Part model, mm, in its own coordinate system. Face numbers are marked on the shaded views. A direction names the side the tool comes from. Round coordinates to 2 decimals unless told otherwise and drop trailing zeros. Write each loop counter-clockwise with the first axis right and the second up, starting at its lowest first coordinate (ties: lowest second). Pieces come first, ordered by that corner, then holes. Notation, with made-up numbers: M 12.25,34.5 L 25.25,34.5 A27 cw 25.25,61.5 Z; hole C 56.5,43 d10. An arc over 180 degrees is marked long. Answer as a JSON object with one key per item and string values. Group by question number.
1. Band-saw the part on D-D, the plane z = -11. Write the cut outline in (x, y).
2. Band-saw the part on C-C, the plane x = 44. Write the cut outline in (y, z) (1 decimal).
3. Band-saw the part on A-A, the plane y = 6.5. Write the cut outline in (x, z) (1 decimal).
4. Which spindle directions (+Z, -Z, +X, -X, +Y, -Y) get a long thin tool onto all of the face, cutting with end or side? Do the marked faces 1 and 2. Say none if no direction does.
5. Band-saw the part on B-B, the plane z = -29.5. Write the cut outline in (x, y).
6. Drill centre lines: line 1 (X direction, y = 8, z = -43); line 2 (Y direction, x = 39.5, z = -35); line 3 (Z direction, x = 22, y = 1). Where is each one in solid material? Low to high. Write a range as from..to.
7. Drop flat-ended pins along their axis: pin 1 (3 mm diameter, centred on x = 11, y = 5, fed in from -Z); pin 2 (0.8 mm diameter, centred on x = 43.5, y = 0.5, fed in from -Z) (3 decimals); pin 3 (4.5 mm diameter, centred on y = 4.29, z = -47.96, fed in from -X); pin 4 (8 mm diameter, centred on x = 13, z = -20, fed in from +Y). Give the stop position or say it passes through.
8. Two-plate mould, pull along X, no slides. Class the marked faces 3, 4 and 5: +X half, -X half, draft (parallel to the pull), parting line (faces both ways), or undercut.
from build123d import *

# Parameters (mm, degrees)
BOSS_EXTRUDE1_DEPTH = 1.5875
SKETCH2_W           = 1.5875
SKETCH2_H           = 22.225
BOSS_EXTRUDE2_DEPTH = 6.985
FILLET1_R           = 3.175
FILLET2_R           = 3.81
HOLE1_D             = 2.8448


with BuildPart() as part:
    # Sketch1 → Boss-Extrude1 (new body)
    with BuildSketch(Plane(origin=(0, 0, 0), x_dir=(1, 0, 0), z_dir=(0, 1, 0))):
        Polygon((8.9535, 28.575), (8.9535, 50.8), (10.541, 50.8), (10.541, 38.1), (40.259, 38.1), (40.259, 50.8), (41.8465, 50.8), (41.8465, 28.575), (50.8, 28.575), (50.8, 0), (0, 0), (0, 28.575), align=None)
    extrude(amount=BOSS_EXTRUDE1_DEPTH)

    # Sketch2 → Boss-Extrude2 (add)
    with BuildSketch(Plane(origin=(0, 1.5875, 0), x_dir=(1, 0, 0), z_dir=(0, 1, 0))):
        with Locations((9.74725, 39.6875)):
            Rectangle(SKETCH2_W, SKETCH2_H)
        with Locations((41.05275, 39.6875)):
            Rectangle(SKETCH2_W, SKETCH2_H)
    extrude(amount=BOSS_EXTRUDE2_DEPTH)

    # Fillet1
    fillet1_edges = [part.edges().sort_by_distance(p)[0] for p in [
        (9.74725, 0, -50.8),
        (41.05275, 0, -50.8),
        (9.74725, 8.5725, -50.8),
        (41.05275, 8.5725, -50.8),
    ]]
    fillet(fillet1_edges, radius=FILLET1_R)

    # Fillet2
    fillet2_edges = [part.edges().sort_by_distance(p)[0] for p in [
        (0, 0.79375, -28.575),
        (50.8, 0.79375, -28.575),
        (50.8, 0.79375, 0),
        (0, 0.79375, 0),
    ]]
    fillet(fillet2_edges, radius=FILLET2_R)

    # Hole1 (through all)
    with Locations(Plane.ZY.offset(-8.9535)):
        with Locations((-47.9552, 4.28625)):
            Hole(HOLE1_D / 2)


solid = part.part
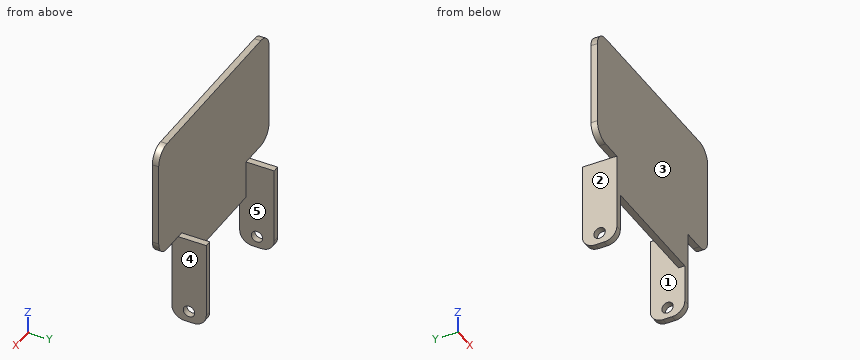
Worked answers:
{
 "1": {"outline": "M 0,0 L 50.8,0 L 50.8,1.59 L 0,1.59 Z"},
 "2": {"outline": "M 0,-28.6 L 1.6,-28.6 L 1.6,0 L 0,0 Z"},
 "3": {"outline": "M 9,-50.6 L 10.5,-50.6 L 10.5,-28.6 L 9,-28.6 Z; M 40.3,-50.6 L 41.8,-50.6 L 41.8,-28.6 L 40.3,-28.6 Z"},
 "4": {"face 1": "-Z, +Y", "face 2": "-Z, -X, +Y, -Y"},
 "5": {"outline": "M 8.95,0 L 41.85,0 L 41.85,8.57 L 40.26,8.57 L 40.26,1.59 L 10.54,1.59 L 10.54,8.57 L 8.95,8.57 Z"},
 "6": {"line 1": "x = 8.95..10.54, 40.26..41.85", "line 2": "y = 0..1.59", "line 3": "z = -38.1..0"},
 "7": {"pin 1": "stops at z = -50.8", "pin 2": "stops at z = -28.575", "pin 3": "stops at x = 8.95", "pin 4": "stops at y = 1.59"},
 "8": {"face 3": "draft", "face 4": "+X half", "face 5": "undercut"}
}
